```python
from build123d import *

# Parameters (mm, degrees)
ESBO_O1_R                = 5.5
RESSALTO_EXTRUS_O1_DEPTH = 22
ESBO_O5_W                = 15
ESBO_O5_H                = 10
CORTE_EXTRUS_O3_DEPTH    = 26
ESBO_O6_R                = 1.5
CORTE_EXTRUS_O4_DEPTH    = 44.548823176


with BuildPart() as part:
    # Esboço1 → Ressalto-extrusão1 (new body)
    with BuildSketch(Plane(origin=(0, 0, 0), x_dir=(0, 0, -1), z_dir=(1, 0, 0))):
        with BuildLine():
            Line((24.5, 0), (7.795898562, 24.754504543))
            ThreePointArc((7.795898562, 24.754504543), (0.921060547, 28.498278549), (-6.098863428, 25.034190078))
            Line((-6.098863428, 25.034190078), (-24.5, 0))
            Line((-24.5, 0), (24.5, 0))
        make_face()
        with Locations((0.75, 20)):
            Circle(ESBO_O1_R, mode=Mode.SUBTRACT)
    extrude(amount=RESSALTO_EXTRUS_O1_DEPTH)

    # Esboço5 → Corte-extrusão3 (cut)
    with BuildSketch(Plane(origin=(0, 28.5, 0), x_dir=(1, 0, 0), z_dir=(0, 1, 0))):
        with Locations((11, 19.5)):
            Rectangle(ESBO_O5_W, ESBO_O5_H)
        with Locations((11, -19.5)):
            Rectangle(ESBO_O5_W, ESBO_O5_H)
    extrude(amount=-CORTE_EXTRUS_O3_DEPTH, mode=Mode.SUBTRACT)

    # Esboço6 → Corte-extrusão4 (cut, through all)
    with BuildSketch(Plane(origin=(0, 28.5, 0), x_dir=(1, 0, 0), z_dir=(0, 1, 0))):
        with Locations(Location((11, 20, 0), (0, 0, 270))):
            Circle(ESBO_O6_R)
        with Locations(Location((11, -20, 0), (0, 0, 270))):
            Circle(ESBO_O6_R)
    extrude(amount=-CORTE_EXTRUS_O4_DEPTH, mode=Mode.SUBTRACT)


solid = part.part
```
Here's how the part is built. I have some questions about the finished solid (model axes, mm). A direction names the side the tool comes from. Give positions to 0.01 mm unless a question says otherwise; leave off trailing zeros. Order: outer loops, then holes, each group sorted by start corner. A loop starts at its lowest first (then second) coordinate and runs counter-clockwise, first axis right, second up. Notation, with made-up numbers: (-5, -27.5) -> (-1, -27.5) arc R27 ccw to (-1, 1.5) -> close; hole circle Ø3 at (54.25, 9). An arc over 180 degrees is marked (long way). Use CSV: the item, a comma, the result in double quotes. Start each with the question number.
Item 1: If I drill on probe 1 along Y at (x, z) = (7.5, -0.75); probe 2 along X at (y, z) = (1, 20); probe 3 along Y at (x, z) = (16.5, 4), over which ranges is the centre line in solid material (lowest first)? Write a range as [from, to].
Item 2: Suppose I cut it at D-D (x = 14.5). List the corners of the cut face in (y, z) for me, and give its area (3 significant figures).
Item 3: Suppose I cut it at A-A (x = 11). List the corners of the cut face in (y, z) for me, and give its area (3 significant figures).
Item 4: On a 3-axis mill with a long thin cutter (end or side, diameter ignored), from which of +Z, -Z, +X, -X, +Y, -Y can I reach the whole of each face in a straight line? I mean faces 1 (the cylindrical face through (11.07, 1.27, 18.5)), 2 (the flat face through (11, 8, 14.5)), 3 (the flat face through (11, 9, -14.5)). Say none if no direction works.
Item 5: Thinking about a two-plate mould opening in Z: for faces 4 (the flat face through (18.5, 6, 17)), 5 (the cylindrical face through (10.846, 25.453, -0.034)), 6 (the cylindrical face through (10.846, 28.495, -1.035)), which applies, pulls with the +Z half, pulls with the -Z half, needs draft (parallel to the pull), parting line crosses it, or undercut?
Item 6: I'm going to push flat-ended pins straight in: P1, Ø4, axis at y = 20.5, z = -13.5, coming from the -X side; P2, Ø8, axis at x = 7, y = 13.5, coming from the -Z side; P3, Ø1, axis at x = 9.5, z = 8, coming from the -Y side; P4, Ø2.5, axis at x = 8.5, z = 18, coming from the +Y side. Where does each tip first touch, or does it pass through?
Item 7: Suppose I cut it at B-B (z = -0.75). List the corners of the cut face in (x, y) for me, and give its area (3 significant figures).
Item 8: Suppose I cut it at C-C (y = 20). List the corners of the cut face in (x, z) for me, and give its area (3 significant figures).
Answer block:
1,probe 1,"y = [0, 14.5], [25.5, 28.5]"
1,probe 2,"x = [0, 9.5], [12.5, 22]"
1,probe 3,"y = [0, 17.23], [22.77, 27.05]"
2,outline,"(0, -24.5) -> (2.5, -22.81) -> (2.5, -14.5) -> (14.82, -14.5) -> (24.75, -7.8) arc R8.5 ccw to (25.03, 6.1) -> (13.6, 14.5) -> (2.5, 14.5) -> (2.5, 22.66) -> (0, 24.5) -> close; hole circle Ø11 at (20, -0.75)"
2,area,"627 mm^2"
3,outline,"(0, -24.5) -> (2.5, -22.81) -> (2.5, -21.5) -> (0, -21.5) -> close; (0, -18.5) -> (2.5, -18.5) -> (2.5, -14.5) -> (14.82, -14.5) -> (24.75, -7.8) arc R8.5 ccw to (25.03, 6.1) -> (13.6, 14.5) -> (2.5, 14.5) -> (2.5, 18.5) -> (0, 18.5) -> close; (0, 21.5) -> (2.5, 21.5) -> (2.5, 22.66) -> (0, 24.5) -> close; hole circle Ø11 at (20, -0.75)"
3,area,"612 mm^2"
4,face 1,"+Y, -Y"
4,face 2,"+Z, +Y"
4,face 3,"-Z, +Y"
5,face 4,"needs draft"
5,face 5,"undercut"
5,face 6,"parting line crosses it"
6,P1,"passes through"
6,P2,"stops at z = -16.7"
6,P3,"stops at y = 0"
6,P4,"stops at y = 2.5"
7,outline,"(0, 0) -> (22, 0) -> (22, 14.5) -> (0, 14.5) -> close; (0, 25.5) -> (22, 25.5) -> (22, 28.5) -> (0, 28.5) -> close"
7,area,"385 mm^2"
8,outline,"(0, -11) -> (22, -11) -> (22, -6.25) -> (0, -6.25) -> close; (0, 4.75) -> (22, 4.75) -> (22, 9.8) -> (0, 9.8) -> close"
8,area,"216 mm^2"
